```python
from build123d import *
from build123d.topology import SkipClean

# Parameters (mm, degrees)
SZKIC1_R                    = 3
DODANIE_WYCI_GNI_CIE1_DEPTH = 2.9
CUT_EXTRUDE1_DEPTH          = 114.129457027
BOSS_EXTRUDE1_START         = -2
BOSS_EXTRUDE1_DEPTH         = 2
SKETCH4_R                   = 7
CUT_EXTRUDE2_DEPTH          = 114.129457027


with BuildPart() as part:
    # Szkic1 → Dodanie-wyciągnięcie1 (new body)
    with BuildSketch(Plane.XY):
        with BuildLine():
            Line((5.59608992, 79.7936944), (5.474471245, 74.546001301))
            ThreePointArc((5.474471245, 74.546001301), (-0.291440696, 69.526456585), (-5.49285922, 75.12885027))
            Line((-5.49285922, 75.12885027), (-5.49285922, 79.844283988))
            ThreePointArc((-5.49285922, 79.844283988), (-14.367089706, 78.768108258), (-23.065888919, 76.708736224))
            Line((-23.065888919, 76.708736224), (-23.039986666, 76.621411569))
            Line((-23.039986666, 76.621411569), (-19.411565048, 68.127477703))
            ThreePointArc((-19.411565048, 68.127477703), (-24.281118736, 54.694699487), (-37.616696357, 59.824461002))
            Line((-37.616696357, 59.824461002), (-41.525713683, 68.39534268))
            Line((-41.525713683, 68.39534268), (-41.581780451, 68.547753974))
            ThreePointArc((-41.581780451, 68.547753974), (-53.538529253, 59.740594559), (-63.661784759, 48.875531428))
            ThreePointArc((-63.661784759, 48.875531428), (-57.63860389, 36.215421703), (-69.476005411, 28.703230861))
            Line((-69.476005411, 28.703230861), (-63.782348494, 26.96242314))
            ThreePointArc((-63.782348494, 26.96242314), (-58.970954639, 18.052629351), (-67.944384326, 13.360988291))
            Line((-67.944384326, 13.360988291), (-78.286081853, 16.522911699))
            Line((-78.286081853, 16.522911699), (-78.582583175, 16.605553861))
            ThreePointArc((-78.582583175, 16.605553861), (-79.500655067, 11.453666872), (-80.079993893, 6.252785978))
            Line((-80.079993893, 6.252785978), (-79.77300326, 6.154050162))
            Line((-79.77300326, 6.154050162), (-74.677344042, 5.483608926))
            ThreePointArc((-74.677344042, 5.483608926), (-69.513002092, -0.180404237), (-75.038066691, -5.493137439))
            Line((-75.038066691, -5.493137439), (-79.77687053, -6.060366735))
            Line((-79.77687053, -6.060366735), (-80.092161675, -6.095570053))
            ThreePointArc((-80.092161675, -6.095570053), (-78.122473499, -18.642914619), (-74.192138812, -30.72049701))
            ThreePointArc((-74.192138812, -30.72049701), (-58.652296854, -33.838462178), (-63.661783627, -48.875530946))
            ThreePointArc((-63.661783627, -48.875530946), (-38.402330015, -70.364141863), (-6.599369234, -79.764784472))
            Line((-6.599369234, -79.764784472), (-6.599369234, -79.734091682))
            Line((-6.599369234, -79.734091682), (-5.427735296, -74.153881943))
            ThreePointArc((-5.427735296, -74.153881943), (0.501919726, -69.539966289), (5.491002421, -75.157624183))
            Line((5.491002421, -75.157624183), (5.357427391, -79.811006311))
            ThreePointArc((5.357427391, -79.811006311), (37.621821152, -70.448066311), (63.198431202, -48.665211389))
            ThreePointArc((63.198431202, -48.665211389), (58.631189133, -33.87502124), (73.70968686, -30.375259673))
            ThreePointArc((73.70968686, -30.375259673), (77.597084263, -18.221882556), (79.503058016, -5.605080347))
            Line((79.503058016, -5.605080347), (75.132623878, -5.498149954))
            ThreePointArc((75.132623878, -5.498149954), (69.518937549, -0.057178034), (75.019100209, 5.498527174))
            Line((75.019100209, 5.498527174), (79.497785184, 5.679667972))
            ThreePointArc((79.497785184, 5.679667972), (77.588561718, 18.258285206), (73.709687487, 30.375260095))
            ThreePointArc((73.709687487, 30.375260095), (58.631189019, 33.875021437), (63.198432292, 48.665211915))
            ThreePointArc((63.198432292, 48.665211915), (59.384670175, 53.274660922), (55.237154752, 57.586263576))
            Line((55.237154752, 57.586263576), (50.019107731, 48.548341019))
            Line((50.019107731, 48.548341019), (38.235772571, 45.391005879))
            Line((38.235772571, 45.391005879), (27.597522321, 26.965015942))
            Line((27.597522321, 26.965015942), (7.360240685, 38.649015942))
            Line((7.360240685, 38.649015942), (17.993490945, 57.066345642))
            Line((17.993490945, 57.066345642), (14.823837521, 68.868339749))
            Line((14.823837521, 68.868339749), (19.653558746, 77.480969916))
            ThreePointArc((19.653558746, 77.480969916), (12.67640031, 78.950827209), (5.59608992, 79.7936944))
        make_face()
        with Locations((-16.270008662, -28.180480518)):
            Circle(SZKIC1_R, mode=Mode.SUBTRACT)
        with Locations((40.540020027, 1.11e-07)):
            Circle(SZKIC1_R, mode=Mode.SUBTRACT)
        with Locations((-19.770010135, 34.242663145)):
            Circle(SZKIC1_R, mode=Mode.SUBTRACT)
    extrude(amount=DODANIE_WYCI_GNI_CIE1_DEPTH)

    # Sketch2 → Cut-Extrude1 (cut, through all)
    with BuildSketch(Plane.XY.offset(2.9)):
        with BuildLine():
            Line((44.364070916, 19.778823857), (13.364070916, -33.914751178))
            Line((13.364070916, -33.914751178), (12.3463525, -33.327171176))
            ThreePointArc((12.3463525, -33.327171176), (3.149700914, -32.090654364), (10.646386774, -26.62191819))
            Line((10.646386774, -26.62191819), (39.167918493, 22.778823857))
            ThreePointArc((39.167918493, 22.778823857), (46.265994705, 29.073052491), (44.364070916, 19.778823857))
        make_face()
        with BuildLine():
            Line((-33.626467493, -6.784751178), (-32.612602806, -7.378895826))
            ThreePointArc((-32.612602806, -7.378895826), (-26.935905927, -14.717570636), (-25.95184679, -5.49191819))
            Line((-25.95184679, -5.49191819), (2.569684929, 43.908823857))
            ThreePointArc((2.569684929, 43.908823857), (4.471608718, 53.203052491), (-2.626467493, 46.908823857))
            Line((-2.626467493, 46.908823857), (-33.626467493, -6.784751178))
        make_face()
    extrude(amount=-CUT_EXTRUDE1_DEPTH, mode=Mode.SUBTRACT)

    # Sketch3 → Boss-Extrude1 (add)
    with SkipClean():  # the faces are left unmerged after this step: merging them gives an invalid solid
        with BuildSketch(Plane(origin=(0, 0, 0), x_dir=(-1, 0, 0), z_dir=(0, 0, -1)).offset(BOSS_EXTRUDE1_START)):
            with BuildLine():
                Line((2.626467493, 46.908823857), (33.626467493, -6.784751178))
                Line((33.626467493, -6.784751178), (32.612602806, -7.378895826))
                ThreePointArc((32.612602806, -7.378895826), (29.661615324, -5.096213752), (25.95184679, -5.49191819))
                Line((25.95184679, -5.49191819), (-2.569684929, 43.908823857))
                ThreePointArc((-2.569684929, 43.908823857), (0.528391282, 44.542798453), (2.626467493, 46.908823857))
            make_face()
            with BuildLine():
                Line((-39.167918493, 22.778823857), (-10.646386774, -26.62191819))
                ThreePointArc((-10.646386774, -26.62191819), (-12.843027181, -29.633130023), (-12.3463525, -33.327171176))
                Line((-12.3463525, -33.327171176), (-13.364070916, -33.914751178))
                Line((-13.364070916, -33.914751178), (-44.364070916, 19.778823857))
                ThreePointArc((-44.364070916, 19.778823857), (-41.265994705, 20.412798453), (-39.167918493, 22.778823857))
            make_face()
        extrude(amount=BOSS_EXTRUDE1_DEPTH)

    # Sketch4 → Cut-Extrude2 (cut, through all)
    with SkipClean():  # the faces are left unmerged after this step: merging them gives an invalid solid
        with BuildSketch(Plane.XY.offset(2.9)):
            with Locations((-34.270008175, -59.357395336)):
                Circle(SKETCH4_R)
            with Locations((57.524732512, -36.364240597)):
                Circle(SKETCH4_R)
        extrude(amount=-CUT_EXTRUDE2_DEPTH, mode=Mode.SUBTRACT)


solid = part.part
```
The model under review builds one solid part; all positions refer to its coordinate system, in mm. A direction names the side the tool comes from. Coordinates: 2 decimals unless noted, no trailing zeros. Write each loop counter-clockwise with the first axis right and the second up, starting at its lowest first coordinate (ties: lowest second). Pieces come first, ordered by that corner, then holes.
1) Machinability: for faces 1 (the face through (-16, 20, 2)), 2 (the face through (32.991, 36.307, 1.43)), 3 (the face through (-78.164, -18.47, 1.43)), which of the approach directions +Z, -Z, +X, -X, +Y, -Y give a long, thin tool a straight path to every point of the face, cutting with its end or side? Answer none if there is none.
2) We need section C-C on z = 1.3. Count the separate pieces of the cut face and the enclosed holes in it, then the cut area to 3 significant figures.
3) The part is to be moulded in two halves that separate along Y. For faces 4 (the face through (-17.91, 20.44, 2.46)), 5 (the face through (59.44, 53.21, 1.43)), 6 (the face through (-38.81, -70.14, 1.43)), say which applies: pulls with the +Y half, pulls with the -Y half, needs draft (parallel to the pull), parting line crosses it, or undercut.
4) We need section D-D on y = 0. State the section outline as (x, z) points.
5) Clearance check with flat-ended pins moving along their axes: pin 1 Ø6 at (x, y) = (28.5, 29) entering from +Z; pin 2 Ø5.5 at (x, y) = (40.54, 0) entering from -Z; pin 3 Ø1 at (x, z) = (-63, 1) entering from -Y; pin 4 Ø1.5 at (x, z) = (35.5, 1) entering from +Y. State where each tip first meets the part, or that it passes through.
6) We need section B-B on y = -62. State the section outline as (x, z) points, then the cut area to 3 significant figures.
7) To check wall thickness, follow probe 1 along Y at (x, z) = (10, 1.9); probe 2 along X at (y, z) = (52, 0.85); probe 3 along Y at (x, z) = (41.5, 1). State the ranges of each line that lie inside material, in increasing order.
8) We need section A-A on y = 25. State the section outline as (x, z) points.
Answer list:
1. face 1: +Z
1. face 2: +Z, -Z, +Y
1. face 3: +Z, -Z, -X, -Y
2. separate pieces: 1
2. enclosed holes: 8
2. area: 16,400 mm2
3. face 4: undercut
3. face 5: pulls with the +Y half
3. face 6: pulls with the -Y half
4. outline: (-69.51, 0) - (37.54, 0) - (37.54, 2.9) - (32.94, 2.9) - (32.94, 2) - (26.02, 2) - (26.02, 2.9) - (-22.78, 2.9) - (-22.78, 2) - (-29.71, 2) - (-29.71, 2.9) - (-69.51, 2.9) - close; (43.54, 0) - (69.52, 0) - (69.52, 2.9) - (43.54, 2.9) - close
5. pin 1: stops at z = 2.9
5. pin 2: passes through
5. pin 3: stops at y = -50.35
5. pin 4: stops at y = 41.95
6. outline: (-50.89, 0) - (-40.75, 0) - (-40.75, 2.9) - (-50.89, 2.9) - close; (-27.79, 0) - (50.26, 0) - (50.26, 2.9) - (-27.79, 2.9) - close
6. area: 256 mm2
7. probe 1: y = -79.34 to -35.44, -26.28 to 37.12, 43.22 to 79.34
7. probe 2: x = -61.12 to -1.93, 5.87 to 15.07, 52.01 to 60.5
7. probe 3: y = -68.22 to -2.84, 2.84 to 20.29, 29.2 to 46.27
8. outline: (-60.58, 0) - (38.77, 0) - (38.77, 2.9) - (-8.35, 2.9) - (-8.35, 2) - (-15.28, 2) - (-15.28, 2.9) - (-60.58, 2.9) - close; (48.76, 0) - (75.69, 0) - (75.69, 2.9) - (48.76, 2.9) - close
